Autodesk Inventor part; units mm, degrees
ref_plane "YZ Plane" through (0, 0, 0) normal (1, 0, 0) x (0, 1, 0)
ref_plane "XZ Plane" through (0, 0, 0) normal (0, 1, 0) x (-1, 0, 0)
ref_plane "XY Plane" through (0, 0, 0) normal (0, 0, 1) x (1, 0, 0)
sketch "Sketch1" plane through (0, 0, 0) normal (0, 0, 1) x (1, 0, 0)
  line L0 (0, 5.9944) -> (6.604, 5.9944)
  line L1 (6.604, 5.9944) -> (6.604, 0)
  line L2 (6.604, 0) -> (0, 0)
  line L3 (0, 0) -> (0, 5.9944)
  dimension "d0" = 5.9944
  dimension "d1" = 6.604
extrude "Extrusion1" add sketch "Sketch1" along normal blind 3.6068
sketch "Sketch2" plane through (0, 0, 3.6068) normal (0, 0, 1) x (1, 0, 0)
  circle A0 centre (3.302, 2.9972) radius 1.7526
  line L0 (6.604, 5.9944) -> (0, 5.9944)
  line L1 (0, 5.9944) -> (0, 0)
  line L2 (0, 0) -> (6.604, 0)
  line L3 (6.604, 0) -> (6.604, 5.9944)
  point P0 (3.302, 5.9944)
  point P1 (6.604, 2.9972)
  dimension "d4" = 3.5052
extrude "Extrusion2" add sketch "Sketch2" along normal blind 0.508 contours A0
properties part number "Button"
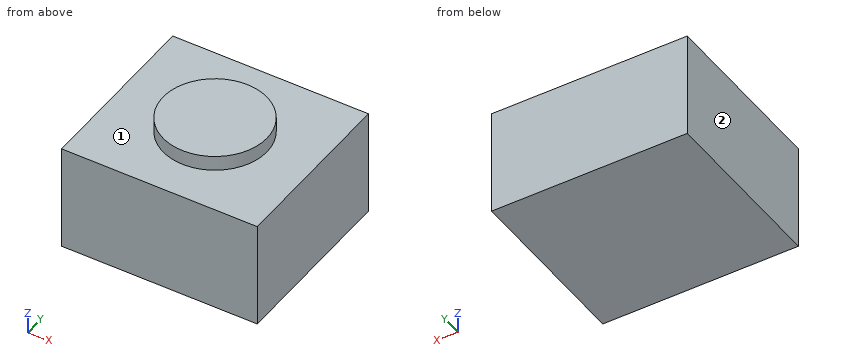
CAD build for the part. Positions are in the model's coordinates, mm. Face numbers are marked on the shaded views. A direction names the side the tool comes from. Coordinates: 2 decimals unless noted, no trailing zeros. Write each loop counter-clockwise with the first axis right and the second up, starting at its lowest first coordinate (ties: lowest second). Pieces come first, ordered by that corner, then holes. Notation, with made-up numbers: (84, 24) -> (90, 24) arc R32 ccw to (90, 59) -> close; hole circle Ø1 at (85.5, 73). An arc over 180 degrees is marked (long way). Return JSON: item names as keys, results as strings. Group by question number.
Q1. Cut at B-B, the plane y = 3.9. Give the cut face in (x, z).
Q2. Cut at A-A, the plane x = 4.25. Give the cut face in (y, z).
Q3. Drill centre lines: line 1 (Z direction, x = 5.5, y = 3.65); line 2 (Y direction, x = 4.75, z = 3.7). Where is each one in solid material? Low to high.
Q4. Flat gauge pin, fed straight in: pin 1 (1 mm diameter, centred on x = 2.5, y = 5, fed in from -Z). Where does the tip first touch, or does it go through?
Q5. Cut at C-C, the plane z = 3.8. Give the cut face in (x, y), then the cut area to 3 significant figures.
Q6. Cut at D-D, the plane y = 5.6. Give the cut face in (x, z).
Q7. Which spindle directions (+Z, -Z, +X, -X, +Y, -Y) get a long thin tool onto all of the face, cutting with end or side? Do the marked faces 1 and 2. Say none if no direction does.
Returned:
{
 "1": {"outline": "(0, 0) -> (6.6, 0) -> (6.6, 3.61) -> (4.8, 3.61) -> (4.8, 4.11) -> (1.8, 4.11) -> (1.8, 3.61) -> (0, 3.61) -> close"},
 "2": {"outline": "(0, 0) -> (5.99, 0) -> (5.99, 3.61) -> (4.47, 3.61) -> (4.47, 4.11) -> (1.52, 4.11) -> (1.52, 3.61) -> (0, 3.61) -> close"},
 "3": {"line 1": "z = 0 to 3.61", "line 2": "y = 2.01 to 3.98"},
 "4": {"pin 1": "stops at z = 0"},
 "5": {"outline": "circle Ø3.51 at (3.3, 3)", "area": "9.65 mm2"},
 "6": {"outline": "(0, 0) -> (6.6, 0) -> (6.6, 3.61) -> (0, 3.61) -> close"},
 "7": {"face 1": "+Z", "face 2": "+Z, -Z, -X, +Y, -Y"}
}
